Verification items for the finished model (mm, model axes). Give positions to 0.01 mm unless a question says otherwise; leave off trailing zeros. Order: outer loops, then holes, each group sorted by start corner. A loop starts at its lowest first (then second) coordinate and runs counter-clockwise, first axis right, second up. Notation, with made-up numbers: (55.5, 5.5) - (104.5, 5.5) arc R12 cw to (104.5, 13.5) - close; hole circle Ø9 at (26, 50). An arc over 180 degrees is marked (long way). Answer as a JSON object with one key per item and string values.
```python
from build123d import *

# Parameters (mm, degrees)
SKETCH1_R           = 12.5
BOSS_EXTRUDE1_DEPTH = 11
BOSS_EXTRUDE2_DEPTH = 22
FILLET1_R           = 10


with BuildPart() as part:
    # Sketch1 → Boss-Extrude1 (new body, symmetric)
    with BuildSketch(Plane.XY):
        with BuildLine():
            Line((-55, 0), (55, 0))
            Line((55, 0), (55, 25))
            Line((55, 25), (28, 25))
            Line((28, 25), (28, 63))
            ThreePointArc((28, 63), (0, 91), (-28, 63))
            Line((-28, 63), (-28, 25))
            Line((-28, 25), (-55, 25))
            Line((-55, 25), (-55, 0))
        make_face()
        with Locations((0, 63)):
            Circle(SKETCH1_R, mode=Mode.SUBTRACT)
    extrude(amount=BOSS_EXTRUDE1_DEPTH, both=True)

    # Sketch2 → Boss-Extrude2 (add)
    with BuildSketch(Plane.XY.offset(11)):
        with BuildLine():
            Line((-55, 25), (-24.101425307, 77.252062944))
            ThreePointArc((-24.101425307, 77.252062944), (-27.007775812, 70.38783092), (-28, 63))
            Line((-28, 63), (-28, 25))
            Line((-28, 25), (-55, 25))
        make_face()
        with BuildLine():
            Line((55, 25), (24.101425307, 77.252062944))
            ThreePointArc((24.101425307, 77.252062944), (27.007775812, 70.38783092), (28, 63))
            Line((28, 63), (28, 25))
            Line((28, 25), (55, 25))
        make_face()
    extrude(amount=-BOSS_EXTRUDE2_DEPTH)

    # Fillet1
    fillet1_edges = [part.edges().sort_by_distance(p)[0] for p in [
        (-55, 25, 0),
        (55, 25, 0),
    ]]
    fillet(fillet1_edges, radius=FILLET1_R)


solid = part.part
```
(1) Section check A-A (z = -7.5). Record the cut outline in (x, y), then the cut area to 3 significant figures.
Computed values:
{"outline": "(-55, 0) - (55, 0) - (55, 22.26) arc R10 ccw to (53.61, 27.35) - (24.1, 77.25) arc R28 ccw to (-24.1, 77.25) - (-53.61, 27.35) arc R10 ccw to (-55, 22.26) - close; hole circle Ø25 at (0, 63)", "area": "6,860 mm²"}
(2) Section check B-B (x = 0). Record the cut outline in (y, z), then the cut area to 3 significant figures.
Computed values:
{"outline": "(0, -11) - (50.5, -11) - (50.5, 11) - (0, 11) - close; (75.5, -11) - (91, -11) - (91, 11) - (75.5, 11) - close", "area": "1,450 mm²"}
(3) Section check D-D (x = 46.5). Record the cut outline in (y, z).
Computed values:
{"outline": "(0, -11) - (39.37, -11) - (39.37, 11) - (0, 11) - close"}
(4) Release check for a two-part mould opening along X. For faces 1 (the flat face through (-55, 11, 0)), 2 (the cylindrical face through (-1.627, 75.394, -0.154)), 3 (the flat face through (1, 36, -11)) record: pulls with the +X half, pulls with the -X half, needs draft (parallel to the pull), parting line crosses it, or undercut.
Computed values:
{"face 1": "pulls with the -X half", "face 2": "undercut", "face 3": "needs draft"}
(5) Gauge pin test, flat end, axial feed: pin 1 Ø12 at (x, z) = (16, 6.5) entering from +Y. Record the tip position at first contact, or that the pin passes through.
Computed values:
{"pin 1": "stops at y = 89.15"}
(6) Material ranges on line 1 along Y through (x, z) = (0, 4); line 2 along Y through (x, z) = (7, 2.75); line 3 along Y through (x, z) = (-46, 8), recorded low to high. Write a range as [from, to].
Computed values:
{"line 1": "y = [0, 50.5], [75.5, 91]", "line 2": "y = [0, 52.64], [73.36, 90.11]", "line 3": "y = [0, 40.22]"}
(7) Section check C-C (y = 58). Record the cut outline in (x, z).
Computed values:
{"outline": "(-35.49, -11) - (-11.46, -11) - (-11.46, 11) - (-35.49, 11) - close; (11.46, -11) - (35.49, -11) - (35.49, 11) - (11.46, 11) - close"}
